Could you check a few things on this model? Use its own coordinates, in mm. A direction names the side the tool comes from. Coordinates: 2 decimals unless noted, no trailing zeros. Loops run counter-clockwise (first coordinate to the right, second up) from the corner with the lowest first, then second, coordinate; pieces in that order, holes last. Notation, with made-up numbers: (-31, 50) -> (27, 50) arc R25 ccw to (27, 78) -> close; hole circle Ø4 at (71.5, 84). An arc over 180 degrees is marked (long way). One line per question, with ' | ' between items.
```python
from build123d import *

# Parameters (mm, degrees)
SKETCH3_R               = 11
SKETCH3_R_2             = 10.2
CUT_EXTRUDE1_REACH      = 188.961
SKETCH4_R               = 3.3
SKETCH5_R               = 3.3
CUT_EXTRUDE2_DEPTH      = 187.960827776
CUT_EXTRUDE3_DEPTH      = 187.960827776
CUT_EXTRUDE3_DEPTH_BACK = 187.960827776


with BuildPart() as part:
    # Sweep2: sweep along a path in Sketch1
    with BuildLine(Plane.XY) as sweep2_path:
        Line((135.278349191, 0), (91.278349191, 0))
        Line((91.278349191, 0), (-91.278349191, 0))
        ThreePointArc((-91.278349191, 0), (-123.018752815, -10.313082304), (-142.635401071, -37.313082304))
        Line((-142.635401071, -37.313082304), (-150.721650809, -62.2))
        Line((-150.721650809, -62.2), (-156.505221402, -80))
    # Sketch3 → Sweep2 (sweep)
    with BuildSketch(Plane(origin=(91.278349191, 0, 0), x_dir=(0, 0, -1), z_dir=(1, 0, 0))):
        Circle(SKETCH3_R)
        Circle(SKETCH3_R_2, mode=Mode.SUBTRACT)
    sweep(path=sweep2_path.line)

    # Sketch4 → Cut-Extrude1 (cut, up to next)
    with BuildSketch(Plane.XY, mode=Mode.PRIVATE) as cut_extrude1_sk1:
        with Locations(Location((-150.721650809, -62.2, 0), (0, 0, 162))):
            Circle(SKETCH4_R)
    cut_extrude1_tool1 = extrude(cut_extrude1_sk1.sketch, amount=CUT_EXTRUDE1_REACH, mode=Mode.PRIVATE) & part.part
    # Sketch4 → Cut-Extrude1 (cut, up to next)
    with BuildSketch(Plane.XY, mode=Mode.PRIVATE) as cut_extrude1_sk2:
        with BuildLine():
            Line((135.282015265, 2.1), (135.282015265, -2.1))
            Line((135.282015265, -2.1), (132.082015265, -2.1))
            ThreePointArc((132.082015265, -2.1), (130.667801703, -1.514213562), (130.082015265, -0.1))
            Line((130.082015265, -0.1), (130.082015265, 0.1))
            ThreePointArc((130.082015265, 0.1), (130.667801703, 1.514213562), (132.082015265, 2.1))
            Line((132.082015265, 2.1), (135.282015265, 2.1))
        make_face()
    cut_extrude1_tool2 = extrude(cut_extrude1_sk2.sketch, amount=CUT_EXTRUDE1_REACH, mode=Mode.PRIVATE) & part.part
    # Sketch4 → Cut-Extrude1 (cut, up to next)
    with BuildSketch(Plane.XY, mode=Mode.PRIVATE) as cut_extrude1_sk3:
        with BuildLine():
            Line((89.778349191, -5), (92.778349191, -5))
            ThreePointArc((92.778349191, -5), (94.192562753, -4.414213562), (94.778349191, -3))
            Line((94.778349191, -3), (94.778349191, 3))
            ThreePointArc((94.778349191, 3), (94.192562753, 4.414213562), (92.778349191, 5))
            Line((92.778349191, 5), (89.778349191, 5))
            ThreePointArc((89.778349191, 5), (88.364135629, 4.414213562), (87.778349191, 3))
            Line((87.778349191, 3), (87.778349191, -3))
            ThreePointArc((87.778349191, -3), (88.364135629, -4.414213562), (89.778349191, -5))
        make_face()
    cut_extrude1_tool3 = extrude(cut_extrude1_sk3.sketch, amount=CUT_EXTRUDE1_REACH, mode=Mode.PRIVATE) & part.part
    add(cut_extrude1_tool1.solids().sort_by_distance((-150.721651, -62.2, 0))[0], mode=Mode.SUBTRACT)
    add(cut_extrude1_tool2.solids().sort_by_distance((132.865722, 0, 0))[0], mode=Mode.SUBTRACT)
    add(cut_extrude1_tool3.solids().sort_by_distance((91.278349, 0, 0))[0], mode=Mode.SUBTRACT)

    # Sketch5 → Cut-Extrude2 (cut, through all)
    with BuildSketch(Plane.XY):
        with Locations(Location((-150.721650809, -62.2, 0), (0, 0, 162))):
            Circle(SKETCH5_R)
    extrude(amount=-CUT_EXTRUDE2_DEPTH, mode=Mode.SUBTRACT)

    # Sketch6 → Cut-Extrude3 (cut, two sides: drawn at the far end of the back side and taken through both)
    with BuildSketch(Plane.XY.offset(-CUT_EXTRUDE3_DEPTH_BACK)):
        with BuildLine():
            Line((130.082015265, 0.1), (130.082015265, -0.1))
            ThreePointArc((130.082015265, -0.1), (130.667801703, -1.514213562), (132.082015265, -2.1))
            Line((132.082015265, -2.1), (135.278349191, -2.1))
            Line((135.278349191, -2.1), (135.278349191, 2.1))
            Line((135.278349191, 2.1), (132.082015265, 2.1))
            ThreePointArc((132.082015265, 2.1), (130.667801703, 1.514213562), (130.082015265, 0.1))
        make_face()
    extrude(amount=CUT_EXTRUDE3_DEPTH + CUT_EXTRUDE3_DEPTH_BACK, mode=Mode.SUBTRACT)


solid = part.part
```
Q1. Imagine slicing it at A-A on z = 3.5. Write out the boundary of the cut face in (x, y).
Values follow:
outline: (-166.42, -76.78) -> (-165.62, -77.04) -> (-151.75, -34.35) arc R63.58 cw to (-91.28, 9.58) -> (135.28, 9.58) -> (135.28, 10.43) -> (-91.28, 10.43) arc R64.43 ccw to (-152.55, -34.09) -> close; (-147.39, -82.96) -> (-146.59, -83.22) -> (-132.72, -40.54) arc R43.57 cw to (-91.28, -10.43) -> (135.28, -10.43) -> (135.28, -9.58) -> (-91.28, -9.58) arc R44.42 ccw to (-133.52, -40.27) -> close
Q2. We'd pull the mould along Y, two halves only. Please class faces 1 (the face through (20.41, 10.74, 2.38)), 2 (the face through (-147.61, -61.1, -10.32)), 3 (the face through (135.278, -10.5, -0.1)): released by +Y, released by -Y, zero draft, split by the parting line, or undercut.
Values follow:
face 1: split by the parting line | face 2: undercut | face 3: zero draft
Q3. Imagine slicing it at B-B on x = 101. Write out the boundary of the cut face in (y, z), plus the area to 3 significant figures.
Values follow:
outline: circle Ø22 at (0, 0); hole circle Ø20.4 at (0, 0) | area: 53.3 mm2
Q4. For faces 4 (the face through (-150.35, -82, 8.1)), 5 (the face through (20.414, 9.049, -4.707)), which set-ups out of +Z, -Z, +X, -X, +Y, -Y let a thin tool reach every point of the face, with its end or its side?
Values follow:
face 4: +Z, -Z, -X, -Y | face 5: +X
Q5. For pin 1 (1 mm diameter, centred on x = 9.5, z = 7, fed in from +Y); pin 2 (1.5 mm diameter, centred on x = 49.5, z = 1.5, fed in from +Y); pin 3 (4 mm diameter, centred on x = -96, z = -1.5, fed in from -Y); pin 4 (8.5 mm diameter, centred on x = -150.72, y = -62.2, fed in from -Z), each with a flat end and sliding along its axis, tell me the tip position at first contact or that it passes through.
Values follow:
pin 1: stops at y = 8.87 | pin 2: stops at y = 10.97 | pin 3: stops at y = -11.48 | pin 4: stops at z = -11
Q6. Please list where these lines run through material, in increasing order: L1, parallel to Z at x = 74.5, y = 0; L2, parallel to Y at x = -21.5, z = 0.75; L3, parallel to X at y = -43, z = 4.25. Write a range as [from, to].
Values follow:
L1: z = [-11, -10.2], [10.2, 11] | L2: y = [-10.97, -10.17], [10.17, 10.97] | L3: x = [-155.15, -154.23], [-134.73, -133.82]
